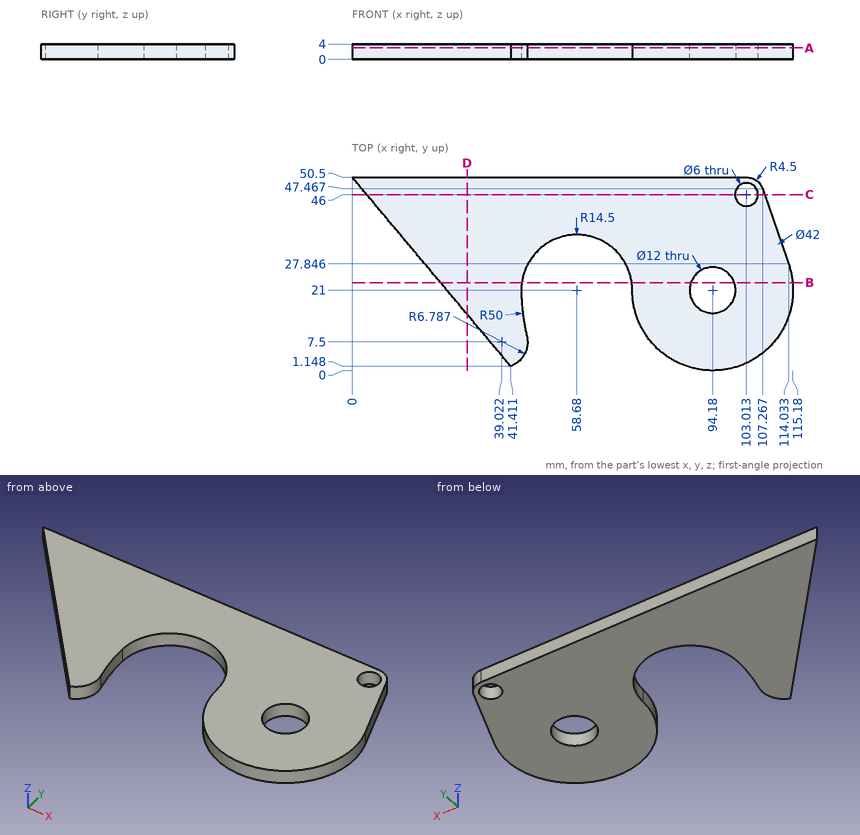
Geometry: see drawing. Coordinates: mm, zero at the bounding-box minimum. Coordinates: 2 decimals unless noted, no trailing zeros. Loops run counter-clockwise (first coordinate to the right, second up) from the corner with the lowest first, then second, coordinate; pieces in that order, holes last. Notation, with made-up numbers: (56, 63) - (71, 63) arc R33 ccw to (71, 96) - close; hole circle Ø9 at (-9.5, -38). An arc over 180 degrees is marked (long way). Answer in a Markdown table with one row per item.
(1) Cut plane D-D on x = 30. Output: boundary loops of the cut face in (y, z), plus the area to 3 significant figures.
Model answer:
| item | result |
|---|---|
| outline | (14.75, 0) - (50.5, 0) - (50.5, 4) - (14.75, 4) - close |
| area | 143 mm² |
(2) Cut plane A-A on z = 3. Output: boundary loops of the cut face in (x, y) (1 decimal), plus the area to 3 significant figures.
Model answer:
| item | result |
|---|---|
| outline | (0, 50.5) - (41.4, 1.1) arc R6.8 ccw to (45.6, 9.1) arc R50 cw to (44.2, 21) arc R14.5 cw to (73.2, 21) arc R21 ccw (long way) to (114, 27.8) - (107.3, 47.5) arc R4.5 ccw to (103, 50.5) - close; hole circle Ø12 at (94.2, 21); hole circle Ø6 at (103, 46) |
| area | 3,370 mm² |
(3) Pin query (flat end, axial travel): P1, Ø1.5, axis at y = 45, z = 3.5, coming from the +X side; P2, Ø1, axis at y = 37.5, z = 2.5, coming from the +X side. Return the tip coordinate at first contact, or that it passes through.
Model answer:
| item | result |
|---|---|
| P1 | stops at x = 108.38 |
| P2 | stops at x = 110.88 |
(4) Cut plane B-B on y = 23. Output: boundary loops of the cut face in (x, z) (1 decimal), plus the area to 3 significant figures.
Model answer:
| item | result |
|---|---|
| outline | (23.1, 0) - (44.3, 0) - (44.3, 4) - (23.1, 4) - close; (73, 0) - (88.5, 0) - (88.5, 4) - (73, 4) - close; (99.8, 0) - (115.1, 0) - (115.1, 4) - (99.8, 4) - close |
| area | 208 mm² |
(5) Cut plane C-C on y = 46. Output: boundary loops of the cut face in (x, z).
Model answer:
| item | result |
|---|---|
| outline | (3.78, 0) - (100.01, 0) - (100.01, 4) - (3.78, 4) - close; (106.01, 0) - (107.77, 0) - (107.77, 4) - (106.01, 4) - close |
(6) Material intervals for L1, parallel to X at y = 17.5, z = 3 (1 decimal); L2, parallel to Y at x = 89.5, z = 1.6 (1 decimal); L3, parallel to X at y = 29.5, z = 3.2 (1 decimal), sorted ascending. Write a range as from..to.
Model answer:
| item | result |
|---|---|
| L1 | x = 27.7..44.3, 73.5..89.3, 99.1..114.9 |
| L2 | y = 0.5..17.2, 24.8..50.5 |
| L3 | x = 17.6..46.9, 70.4..113.5 |
